The model under review builds one solid part; all positions refer to its coordinate system, in mm. A direction names the side the tool comes from. Round coordinates to 2 decimals unless told otherwise and drop trailing zeros. Loops run counter-clockwise (first coordinate to the right, second up) from the corner with the lowest first, then second, coordinate; pieces in that order, holes last. Notation, with made-up numbers: M -2.75,38 L 42.25,38 A17 cw 42.25,55 Z; hole C 31.5,-37.75 d10. An arc over 180 degrees is marked long. Answer as a JSON object with one key per item and string values. Group by question number.
Item 1: Consider section D-D (y = -11.25). Give the boundary of the cut face in (x, z).
Item 2: Consider section B-B (y = 0). Give the boundary of the cut face in (x, z).
Item 3: Consider section A-A (z = 0.4). Give the boundary of the cut face in (x, y).
Item 4: Tool access review of faces 1 (the face through (4, -7, 2)), 2 (the face through (9.9, 0, 1)): name each direction out of +Z, -Z, +X, -X, +Y, -Y from which nothing blocks a thin tool from reaching the whole face with its end or side.
Item 5: The part is to be moulded in two halves that separate along Y. For faces 3 (the face through (4, -20, 1)), 4 (the face through (-5, -8, 1)), 5 (the face through (4.9, -10, 1)), say which applies: +Y half, -Y half, draft (parallel to the pull), parting line (faces both ways), or undercut.
Item 6: Insertion check: P1, Ø5, axis at x = 0, y = 0, coming from the +Z side. The pin has a flat end and moves straight along its axis. Give the tip position at first contact, or say it passes through.
Item 7: Consider section C-C (x = 5.25). Give the boundary of the cut face in (y, z).
Item 8: To check wall thickness, follow line 1 (Y direction, x = 0, z = 1.1); line 2 (X direction, y = 1.75, z = 1.95); line 3 (Y direction, x = -1, z = 1.4). State the ranges of each line that lie inside material, in increasing order.
```python
from build123d import *

# Parameters (mm, degrees)
SKETCH_W      = 17.8
SKETCH_H      = 25
SKETCH_R      = 2.1
EXTRUDE_DEPTH = 2


with BuildPart() as part:
    # Sketch → Extrude (new body)
    with BuildSketch(Plane.XY):
        with Locations((3.9, -7.5)):
            Rectangle(SKETCH_W, SKETCH_H)
        Circle(SKETCH_R, mode=Mode.SUBTRACT)
        with Locations((0, -15)):
            Circle(SKETCH_R, mode=Mode.SUBTRACT)
        with Locations((0, -10)):
            Circle(SKETCH_R, mode=Mode.SUBTRACT)
        with BuildLine():
            ThreePointArc((7, 2.1), (4.9, 0), (7, -2.1))
            Line((7, -2.1), (7.8, -2.1))
            ThreePointArc((7.8, -2.1), (9.9, 0), (7.8, 2.1))
            Line((7, 2.1), (7.8, 2.1))
        make_face(mode=Mode.SUBTRACT)
        with BuildLine():
            ThreePointArc((7, -12.9), (4.9, -15), (7, -17.1))
            Line((7, -17.1), (7.8, -17.1))
            ThreePointArc((7.8, -17.1), (9.9, -15), (7.8, -12.9))
            Line((7, -12.9), (7.8, -12.9))
        make_face(mode=Mode.SUBTRACT)
        with BuildLine():
            ThreePointArc((7, -7.9), (4.9, -10), (7, -12.1))
            Line((7, -12.1), (7.8, -12.1))
            ThreePointArc((7.8, -12.1), (9.9, -10), (7.8, -7.9))
            Line((7, -7.9), (7.8, -7.9))
        make_face(mode=Mode.SUBTRACT)
    extrude(amount=EXTRUDE_DEPTH)


solid = part.part
```
Geometry results:
{
 "1": {"outline": "M -5,0 L -1.69,0 L -1.69,2 L -5,2 Z; M 1.69,0 L 5.31,0 L 5.31,2 L 1.69,2 Z; M 9.49,0 L 12.8,0 L 12.8,2 L 9.49,2 Z"},
 "2": {"outline": "M -5,0 L -2.1,0 L -2.1,2 L -5,2 Z; M 2.1,0 L 4.9,0 L 4.9,2 L 2.1,2 Z; M 9.9,0 L 12.8,0 L 12.8,2 L 9.9,2 Z"},
 "3": {"outline": "M -5,-20 L 12.8,-20 L 12.8,5 L -5,5 Z; hole C 0,-15 d4.2; hole C 0,-10 d4.2; hole C 0,0 d4.2; hole M 7,-17.1 L 7.8,-17.1 A2.1 ccw 7.8,-12.9 L 7,-12.9 A2.1 ccw Z; hole M 7,-12.1 L 7.8,-12.1 A2.1 ccw 7.8,-7.9 L 7,-7.9 A2.1 ccw Z; hole M 7,-2.1 L 7.8,-2.1 A2.1 ccw 7.8,2.1 L 7,2.1 A2.1 ccw Z"},
 "4": {"face 1": "+Z, +X, -X, +Y, -Y", "face 2": "+Z, -Z"},
 "5": {"face 3": "-Y half", "face 4": "draft", "face 5": "undercut"},
 "6": {"P1": "stops at z = 2"},
 "7": {"outline": "M -20,0 L -16.16,0 L -16.16,2 L -20,2 Z; M -13.84,0 L -11.16,0 L -11.16,2 L -13.84,2 Z; M -8.84,0 L -1.16,0 L -1.16,2 L -8.84,2 Z; M 1.16,0 L 5,0 L 5,2 L 1.16,2 Z"},
 "8": {"line 1": "y = -20 to -17.1, -12.9 to -12.1, -7.9 to -2.1, 2.1 to 5", "line 2": "x = -5 to -1.16, 1.16 to 5.84, 8.96 to 12.8", "line 3": "y = -20 to -16.85, -13.15 to -11.85, -8.15 to -1.85, 1.85 to 5"}
}
